Here's how the part is built. I have some questions about the finished solid (model axes, mm). A direction names the side the tool comes from. Round coordinates to 2 decimals unless told otherwise and drop trailing zeros. Answer in a Markdown table with one row per item. Add a question column.
from build123d import *

# Parameters (mm, degrees)
SKETCH1_W                            = 47.625
SKETCH1_H                            = 63.5
CUT_EXTRUDE1_REACH                   = 94.906
CUT_EXTRUDE1_DIRECTION_2_REACH       = 94.906
SKETCH5_R                            = 23.8125
SKETCH5_R_2                          = 13.49375
BOSS_EXTRUDE1_DEPTH                  = 12.7
BOSS_EXTRUDE1_DIRECTION_2_REACH      = 145.973
BOSS_EXTRUDE1_DIRECTION_2_END_RADIUS = 63.5
CUT_EXTRUDE6_DEPTH                   = 7.9375


with BuildPart() as part:
    # Sketch1 → Revolve1 (revolve)
    with BuildSketch(Plane(origin=(0, 0, 0), x_dir=(0, 0, -1), z_dir=(1, 0, 0)), mode=Mode.PRIVATE) as revolve1_sk:
        with Locations((0, 31.75)):
            Rectangle(SKETCH1_W, SKETCH1_H)
    revolve(revolve1_sk.sketch.rotate(Axis((0, 0, 23.8125), (0, 0, -1)), 90), axis=Axis((0, 0, 23.8125), (0, 0, -1)))

    # Sketch2 → Cut-Extrude1 (cut, up to next)
    with BuildSketch(Plane(origin=(0, 0, 0), x_dir=(0, 0, -1), z_dir=(1, 0, 0)), mode=Mode.PRIVATE) as cut_extrude1_sk1:
        Polygon((-12.7, -63.5), (-23.8125, 63.5), (-23.8125, -63.5), align=None)
    cut_extrude1_tool1 = extrude(cut_extrude1_sk1.sketch, amount=-CUT_EXTRUDE1_REACH, mode=Mode.PRIVATE) & part.part
    # Sketch2 → Cut-Extrude1 (cut, up to next)
    with BuildSketch(Plane(origin=(0, 0, 0), x_dir=(0, 0, -1), z_dir=(1, 0, 0)), mode=Mode.PRIVATE) as cut_extrude1_sk2:
        Polygon((23.8125, 63.5), (12.7, -63.5), (23.8125, -63.5), align=None)
    cut_extrude1_tool2 = extrude(cut_extrude1_sk2.sketch, amount=-CUT_EXTRUDE1_REACH, mode=Mode.PRIVATE) & part.part
    add(cut_extrude1_tool1.solids().sort_by_distance((0, -21.166667, 20.108333))[0], mode=Mode.SUBTRACT)
    add(cut_extrude1_tool2.solids().sort_by_distance((0, -21.166667, -20.108333))[0], mode=Mode.SUBTRACT)

    # Sketch2 → Cut-Extrude1 direction 2 (cut, up to next)
    with BuildSketch(Plane(origin=(0, 0, 0), x_dir=(0, 0, -1), z_dir=(1, 0, 0)), mode=Mode.PRIVATE) as cut_extrude1_direction_2_sk1:
        Polygon((-12.7, -63.5), (-23.8125, 63.5), (-23.8125, -63.5), align=None)
    cut_extrude1_direction_2_tool1 = extrude(cut_extrude1_direction_2_sk1.sketch, amount=CUT_EXTRUDE1_DIRECTION_2_REACH, mode=Mode.PRIVATE) & part.part
    # Sketch2 → Cut-Extrude1 direction 2 (cut, up to next)
    with BuildSketch(Plane(origin=(0, 0, 0), x_dir=(0, 0, -1), z_dir=(1, 0, 0)), mode=Mode.PRIVATE) as cut_extrude1_direction_2_sk2:
        Polygon((23.8125, 63.5), (12.7, -63.5), (23.8125, -63.5), align=None)
    cut_extrude1_direction_2_tool2 = extrude(cut_extrude1_direction_2_sk2.sketch, amount=CUT_EXTRUDE1_DIRECTION_2_REACH, mode=Mode.PRIVATE) & part.part
    add(cut_extrude1_direction_2_tool1.solids().sort_by_distance((0, -21.166667, 20.108333))[0], mode=Mode.SUBTRACT)
    add(cut_extrude1_direction_2_tool2.solids().sort_by_distance((0, -21.166667, -20.108333))[0], mode=Mode.SUBTRACT)

    # Sketch3 → Cut-Revolve1 (revolve, cut)
    with BuildSketch(Plane(origin=(0, 0, 0), x_dir=(0, 0, -1), z_dir=(1, 0, 0))):
        Polygon((-14.093252917, -47.577109525), (-13.828168926, -50.606640849), (-10.288822106, -49.658275727), (-10.288822106, -46.557715362), align=None)
        Polygon((-13.552471291, -53.757470955), (-13.274658791, -56.932470955), (-10.288822106, -57.732523484), (-10.288822106, -54.631963119), align=None)
    revolve(axis=Axis((0, 0, 18.25625), (0, 0.08716695028091019, -0.9961937174961131)), mode=Mode.SUBTRACT)

    # Sketch3<4> → Cut-Revolve2 (revolve, cut)
    with BuildSketch(Plane(origin=(0, 0, 0), x_dir=(0, 0, -1), z_dir=(1, 0, 0)), mode=Mode.PRIVATE) as cut_revolve2_sk:
        Polygon((13.274658791, -56.932470955), (13.552471291, -53.757470955), (10.288822106, -54.631963119), (10.288822106, -57.732523484), align=None)
        Polygon((14.093252917, -47.577109525), (10.288822106, -46.557715362), (10.288822106, -49.658275727), (13.828168926, -50.606640849), align=None)
    revolve(cut_revolve2_sk.sketch.rotate(Axis((0, 0, -18.25625), (0, 0.08716695028091019, 0.9961937174961131)), 180), axis=Axis((0, 0, -18.25625), (0, 0.08716695028091019, 0.9961937174961131)), mode=Mode.SUBTRACT)

    # Sketch4 → Cut-Revolve3 (revolve, cut)
    with BuildSketch(Plane(origin=(0, 0, 0), x_dir=(0, 0, -1), z_dir=(1, 0, 0))):
        with BuildLine():
            Line((0, 63.5), (0, -63.5))
            Line((0, -63.5), (-9.525, -63.5))
            Line((-9.525, -63.5), (-6.35, -60.325))
            Line((-6.35, -60.325), (-6.35, -46.667360082))
            Line((-6.35, -46.667360082), (-7.9375, -45.079860082))
            Line((-7.9375, -45.079860082), (-15.65055133, 43.069297973))
            ThreePointArc((-15.65055133, 43.069297973), (-15.321732353, 44.037994297), (-14.385385309, 44.45))
            Line((-14.385385309, 44.45), (-13.49375, 44.45))
            Line((-13.49375, 44.45), (-13.49375, 76.2))
            Line((-13.49375, 76.2), (0, 76.2))
            Line((0, 76.2), (0, 63.5))
        make_face()
    revolve(axis=Axis((0, 63.5, 0), (0, -1, 0)), mode=Mode.SUBTRACT)


with BuildPart() as boss_extrude1_tool:
    # Sketch5 → Boss-Extrude1 (new body)
    with BuildSketch(Plane(origin=(0, 63.5, 0), x_dir=(1, 0, 0), z_dir=(0, 1, 0))):
        with Locations(Location((0, 0, 0), (0, 0, 270))):
            Circle(SKETCH5_R)
        with Locations(Location((0, 0, 0), (0, 0, 270))):
            Circle(SKETCH5_R_2, mode=Mode.SUBTRACT)
    extrude(amount=BOSS_EXTRUDE1_DEPTH)


with BuildPart() as part_1:
    add(part.part)


with BuildPart() as part_2:
    # Boss-Extrude1: joined with boss_extrude1_tool
    add(part_1.part.fuse(boss_extrude1_tool.part, tol=0.00001))

    # Boss-Extrude1 direction 2: up to this cylinder (the profile starts outside it)
    boss_extrude1_direction_2_end = Plane(origin=(0, 0, -23.138981), z_dir=(0, 0, 1)) * Cylinder(BOSS_EXTRUDE1_DIRECTION_2_END_RADIUS, 419.946, mode=Mode.PRIVATE)
    # Sketch5 → Boss-Extrude1 direction 2 (add, up to the surface)
    with BuildSketch(Plane(origin=(0, 63.5, 0), x_dir=(1, 0, 0), z_dir=(0, 1, 0)), mode=Mode.PRIVATE) as boss_extrude1_direction_2_sk1:
        with Locations(Location((0, 0, 0), (0, 0, 270))):
            Circle(SKETCH5_R)
        with Locations(Location((0, 0, 0), (0, 0, 270))):
            Circle(SKETCH5_R_2, mode=Mode.SUBTRACT)
    boss_extrude1_direction_2_tool1 = extrude(boss_extrude1_direction_2_sk1.sketch, amount=-BOSS_EXTRUDE1_DIRECTION_2_REACH, mode=Mode.PRIVATE) - boss_extrude1_direction_2_end
    add(boss_extrude1_direction_2_tool1.solids().sort_by_distance((0, 63.5, -23.138981))[0])
    add(boss_extrude1_direction_2_tool1.solids().sort_by_distance((0, 63.5, -23.138981))[1])

    # Sketch6 → Cut-Extrude6 (cut, symmetric)
    with BuildSketch(Plane.XY):
        Polygon((0, 27.783421303), (0, -50.606640849), (6.35, -50.401562476), (6.35, -46.667360082), (7.9375, -45.079860082), (14.313037121, 27.783421303), align=None)
        with BuildLine():
            ThreePointArc((28.548758758, -42.01914294), (17.945670231, -47.524655916), (6.35, -50.401562476))
            Line((6.35, -50.401562476), (6.35, -46.667360082))
            Line((6.35, -46.667360082), (7.9375, -45.079860082))
            Line((7.9375, -45.079860082), (14.313037121, 27.783421303))
            Line((14.313037121, 27.783421303), (37.658075276, 51.128459458))
            Line((37.658075276, 51.128459458), (46.638331397, 60.108715579))
            Line((46.638331397, 60.108715579), (60.108715579, 46.638331397))
            Line((60.108715579, 46.638331397), (51.128459458, 37.658075276))
            Line((51.128459458, 37.658075276), (44.74493597, 31.274551788))
            ThreePointArc((44.74493597, 31.274551788), (44.056682484, 30.244507656), (43.815, 29.029487758))
            Line((43.815, 29.029487758), (43.815, 25.425127265))
            ThreePointArc((43.815, 25.425127265), (43.279916019, 23.661191775), (41.855019898, 22.491809749))
            Line((41.855019898, 22.491809749), (32.467470153, 18.603359327))
            ThreePointArc((32.467470153, 18.603359327), (29.890023726, 12.380853207), (36.112529847, 9.80340678))
            Line((36.112529847, 9.80340678), (39.424980102, 11.175468601))
            ThreePointArc((39.424980102, 11.175468601), (42.40393549, 10.882067104), (43.815, 8.242151085))
            Line((43.815, 8.242151085), (43.815, -8.242151085))
            ThreePointArc((43.815, -8.242151085), (42.40393549, -10.882067104), (39.424980102, -11.175468601))
            Line((39.424980102, -11.175468601), (36.112529847, -9.80340678))
            ThreePointArc((36.112529847, -9.80340678), (29.890023726, -12.380853207), (32.467470153, -18.603359327))
            Line((32.467470153, -18.603359327), (41.855019898, -22.491809749))
            ThreePointArc((41.855019898, -22.491809749), (43.279916019, -23.661191775), (43.815, -25.425127265))
            Line((43.815, -25.425127265), (43.815, -29.029487758))
            ThreePointArc((43.815, -29.029487758), (44.056682484, -30.244507656), (44.74493597, -31.274551788))
            Line((44.74493597, -31.274551788), (51.128459458, -37.658075276))
            Line((51.128459458, -37.658075276), (60.108715579, -46.638331397))
            Line((60.108715579, -46.638331397), (46.638331397, -60.108715579))
            Line((46.638331397, -60.108715579), (37.658075276, -51.128459458))
            Line((37.658075276, -51.128459458), (28.548758758, -42.01914294))
        make_face()
        with BuildLine():
            ThreePointArc((15.08125, -22.225), (19.05, -26.19375), (23.01875, -22.225))
            Line((23.01875, -22.225), (23.01875, 22.225))
            ThreePointArc((23.01875, 22.225), (19.05, 26.19375), (15.08125, 22.225))
            Line((15.08125, 22.225), (15.08125, -22.225))
        make_face(mode=Mode.SUBTRACT)
        with BuildLine():
            ThreePointArc((53.34, -34.454236314), (63.5, 0), (53.34, 34.454236314))
            Line((53.34, 34.454236314), (53.34, -34.454236314))
        make_face()
    extrude(amount=CUT_EXTRUDE6_DEPTH, both=True, mode=Mode.SUBTRACT)


solid = part_2.part
Item 1: On a 3-axis mill with a long thin cutter (end or side, diameter ignored), from which of +Z, -Z, +X, -X, +Y, -Y can I reach the whole of each face in a straight line? I mean faces 4 (the flat face through (15.081, 0, 0)), 5 (the flat face through (23.815, -52.037, 13.703)), 6 (the cylindrical face through (43.265, -23.639, -0.111)), 7 (the flat face through (57, 0, 7.938)), 8 (the conical face through (52.734, 11.679, 19.123)). Say none if no direction works.
Item 2: If we mould it in two halves opening along Y, with no side actions, what happens to faces 1 (the conical face through (-6.624, -46.392, 0.146)), 2 (the flat face through (47.715, -19.659, -16.536)), 3 (the flat face through (25, -11, 7.938))? For each: pulls with the +Y half, pulls with the -Y half, needs draft (parallel to the pull), parting line crosses it, or undercut.
Item 3: If we section it at A-A on x = 34.29: Give the number of separate pieces and of enclosed holes in the cut face, then the cut area to 3 significant figures.
Item 4: I need wall thicknesses on line 1 along Z through (x, y) = (0, -56.75); line 2 along Y through (x, z) = (-26, 12); line 3 along X through (y, z) = (71.75, 0). Which ranges of each line are inside material? Lowest first, please. Write a range as from..to.
Item 5: For P1, Ø12, axis at x = 46, z = -6, coming from the +Y side; P2, Ø1.7, axis at y = -47, z = 7, coming from the +X side; P3, Ø10, axis at y = -17.5, z = 11.5, coming from the -X side, each with a flat end and sliding along its axis, tell me the tip position at first contact or that it passes through.
Results list:
| question | item | result |
|---|---|---|
| 1 | face 4 | none |
| 1 | face 5 | +Z, +X, -X, -Y |
| 1 | face 6 | -Y |
| 1 | face 7 | +X, +Y, -Y |
| 1 | face 8 | +Z |
| 2 | face 1 | pulls with the +Y half |
| 2 | face 2 | pulls with the -Y half |
| 2 | face 3 | undercut |
| 3 | separate pieces | 1 |
| 3 | enclosed holes | 3 |
| 3 | area | 2,590 mm² |
| 4 | line 1 | -10.29..-6.35, 6.35..10.29 |
| 4 | line 2 | -57.93..-51.26, -47.78..-42.74, -39.07..57.93 |
| 4 | line 3 | -23.81..-13.49, 13.49..23.81 |
| 5 | P1 | y = 49.06 |
| 5 | P2 | x = 34.38 |
| 5 | P3 | x = -62.26 |
